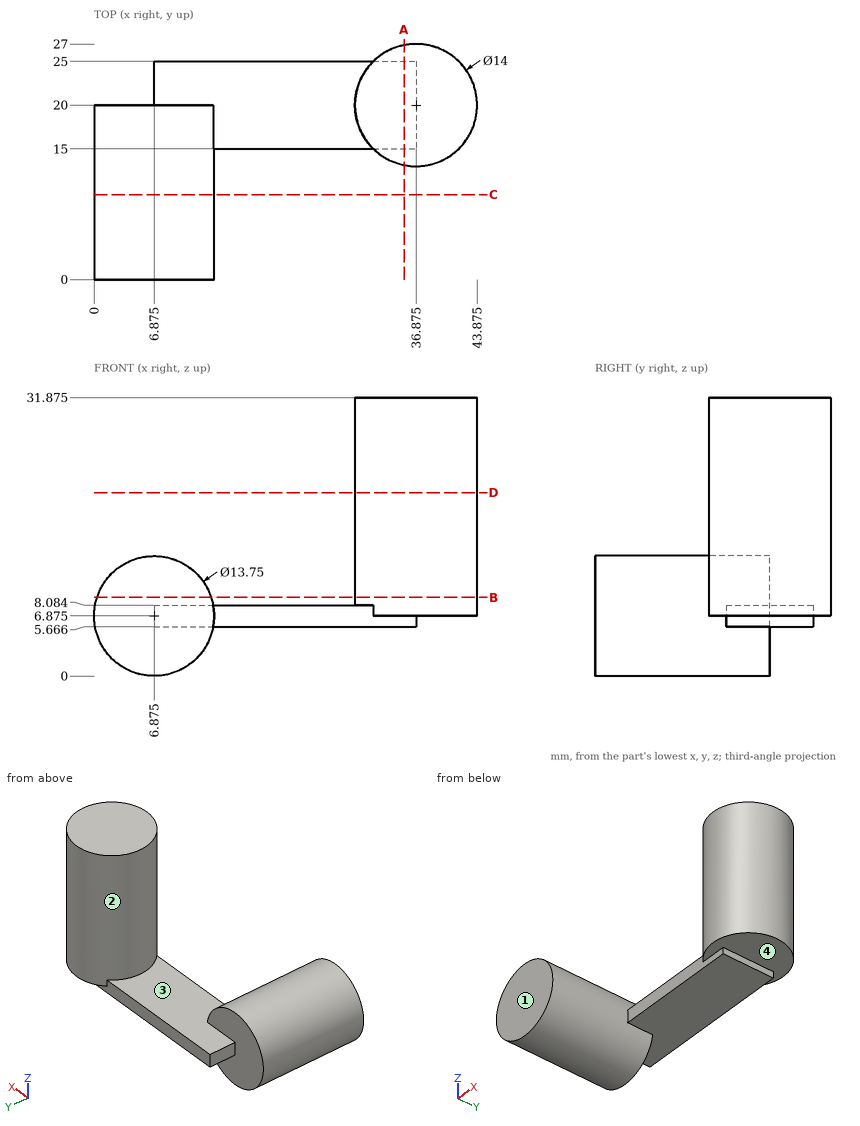
The drawing under review shows one solid part. Ordinate dimensions are in mm from its lowest x, y, z. A direction names the side the tool comes from. Coordinates: 2 decimals unless noted, no trailing zeros. Write each loop counter-clockwise with the first axis right and the second up, starting at its lowest first coordinate (ties: lowest second). Pieces come first, ordered by that corner, then holes. Notation, with made-up numbers: (-38.5, 4) - (-0.5, 4) arc R33 ccw to (-0.5, 36) - close; hole circle Ø5 at (81.25, 82.5). An arc over 180 degrees is marked (long way). Put each result on its own line as item: value.
1. For pin 1 (1.5 mm diameter, centred on x = 33, y = 19, fed in from -Z); pin 2 (0.6 mm diameter, centred on y = 21, z = 6, fed in from +X) (3 decimals); pin 3 (15 mm diameter, centred on x = 7.5, z = 6, fed in from +Y); pin 4 (3 mm diameter, centred on x = 26.5, z = 17.5, fed in from -Y), all flat-tipped, find the tip position at first contact; note any pin that passes through.
Values found:
pin 1: z = 5.67
pin 2: x = 36.875
pin 3: y = 25
pin 4: through
2. Mouldability with a two-part tool opening along X and no side actions: class the marked faces 3 and 4 as released by +X, released by -X, zero draft, split by the parting line, or undercut.
Values found:
face 3: undercut
face 4: zero draft
3. Add section D-D, the plane z = 21. Give the boundary of the cut face in (x, y) (3 decimals).
Values found:
outline: circle Ø14 at (36.875, 20)
4. Wall thickness on probe 1 along Y at (x, z) = (14, 8); probe 2 along Z at (x, y) = (41, 23.5) (3 decimals); probe 3 along Y at (x, z) = (12.5, 9): over which ranges is each line inside the solid? List them lowest first.
Values found:
probe 1: 15 to 25
probe 2: 6.875 to 31.875
probe 3: 0 to 20
5. Add section A-A, the plane x = 35.5. Give the boundary of the cut face in (y, z) (1 decimal).
Values found:
outline: (13.1, 6.9) - (15, 6.9) - (15, 5.7) - (25, 5.7) - (25, 6.9) - (26.9, 6.9) - (26.9, 31.9) - (13.1, 31.9) - close
6. Machinability: for the marked faces 1 and 2, which of the approach directions +Z, -Z, +X, -X, +Y, -Y give a long, thin tool a straight path to every point of the face, cutting with its end or side? Answer none if there is none.
Values found:
face 1: +Z, -Z, +X, -X, -Y
face 2: +Z
7. Add section C-C, the plane y = 9.75. Give the boundary of the cut face in (x, z) (3 decimals).
Values found:
outline: circle Ø13.75 at (6.875, 6.875)
8. Add section B-B, the plane z = 9. Give the boundary of the cut face in (x, y) (1 decimal).
Values found:
outline: (0.3, 0) - (13.4, 0) - (13.4, 20) - (0.3, 20) - close; circle Ø14 at (36.9, 20)
